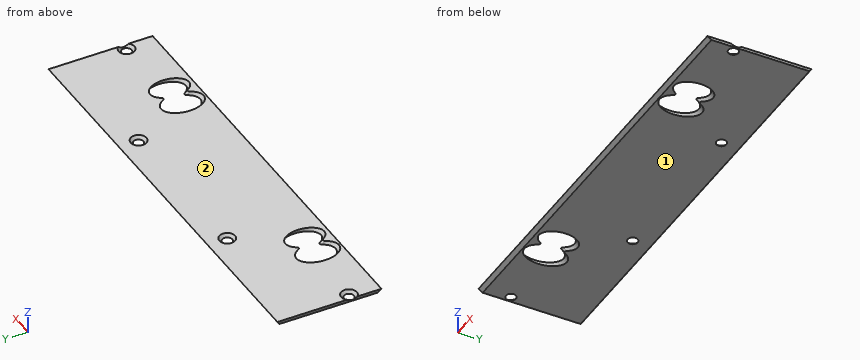
Autodesk Inventor part; units mm, degrees
ref_plane "Work Plane2" through (178, -42.7329, -77.104) normal (1, 0, 0) x (0, 0.819152, -0.5735764)
ref_plane "YZ Plane" through (0, 0, 0) normal (1, 0, 0) x (0, 1, 0)
ref_plane "XZ Plane" through (0, 0, 0) normal (0, 1, 0) x (-1, 0, 0)
ref_plane "Work Plane1" through (0, -45.8455, -0.8595) normal (-1, 0, 0) x (0, 0.5735764, 0.819152)
sketch "Sketch1" plane through (0, -45.8455, -0.8595) normal (-1, 0, 0) x (0, 0.5735764, 0.819152)
  line L0 (4.2002, 4.5) -> (27, 37.0615)
  line L1 (3.5, -0.5) -> (3.5, 3.5)
  line L2 (27, 37.0615) -> (28, 37.0615)
  line L3 (27, 37.0615) -> (3.5, 3.5)
  line L4 (3.5, 1.4079) -> (28.4649, 37.0615)
  line L5 (27, 37.0615) -> (28.4649, 37.0615)
  point P0 (4.2002, 4.5)
  dimension "d0" = 1.2
  dimension "d1" = 55
ref_plane "Work Plane2" through (178, -42.7329, -77.104) normal (1, 0, 0) x (0, 0.819152, -0.5735764)
extrude "Extrusion1" add sketch "Sketch1" against normal up to surface (178 mm away)
ref_plane "Work Plane3" through (36.3849, -23.4357, -7.1547) normal (0, -0.7489557, 0.66262) x (1, 0, 0)
ref_plane "Work Plane4" through (36.3849, -23.4357, -7.1547) normal (0, -0.7489557, 0.66262) x (1, 0, 0)
sketch "Sketch4" plane through (36.3849, -23.4357, -7.1547) normal (0, -0.7489557, 0.66262) x (1, 0, 0)
  line L0 (-14.9215, 5.4518) -> (-14.9215, -5.4534)
  spline S0 degree 3 poles (-14.9215, -5.4534) (-14.9222, -5.5772) (-14.8715, -5.6989) (-14.7851, -5.7853) (-14.7653, -5.8051) (-14.7437, -5.823) (-14.7206, -5.8388) (-14.7012, -5.8521) (-14.6808, -5.864) (-14.6595, -5.8743) (-14.6436, -5.882) (-14.6272, -5.8889) (-14.6105, -5.8948) (-14.5603, -5.9125) (-14.5071, -5.9218) (-14.4534, -5.9215) knots 0 0 0 0 0.5 0.5 0.5 0.614375 0.614375 0.614375 0.710781 0.710781 0.710781 0.783086 0.783086 0.783086 1 1 1 1
  line L1 (-14.4534, -5.9215) -> (14.4534, -5.9215)
  spline S1 degree 3 poles (14.4534, -5.9215) (14.5775, -5.9222) (14.6994, -5.8713) (14.8723, -5.6977) (14.9222, -5.5758) (14.9215, -5.4518) knots 0 0 0 0 0.5 0.5 1 1 1 1
  line L2 (14.9215, -5.4518) -> (14.9215, 5.4534)
  spline S2 degree 3 poles (14.9215, 5.4534) (14.9222, 5.5775) (14.8713, 5.6994) (14.6977, 5.8723) (14.5758, 5.9222) (14.4518, 5.9215) knots 0 0 0 0 0.5 0.5 1 1 1 1
  line L3 (14.4518, 5.9215) -> (-14.4534, 5.9215)
  spline S3 degree 3 poles (-14.4534, 5.9215) (-14.5775, 5.9222) (-14.6994, 5.8713) (-14.8723, 5.6977) (-14.9222, 5.5758) (-14.9215, 5.4518) knots 0 0 0 0 0.5 0.5 1 1 1 1
  circle A0 centre (-13.3791, -4.3791) radius 0.5
  circle A1 centre (-13.3791, 4.3791) radius 0.5
  circle A2 centre (13.3791, 4.3791) radius 0.5
  circle A3 centre (13.3791, -4.3791) radius 0.5
  arc A4 (0.2617, -1.4512) -> (0.1811, -1.5218) centre (0.2771, -1.55) ccw
  arc A5 (0.1811, 1.5218) -> (0.1811, -1.5218) centre (-5, 0) ccw
  arc A6 (0.1811, 1.5218) -> (0.2617, 1.4512) centre (0.2771, 1.55) ccw
  arc A7 (0.2617, 1.4512) -> (0.3414, 1.519) centre (0.2463, 1.55) ccw
  arc A8 (0.3414, -1.519) -> (0.3414, 1.519) centre (5, 0) ccw
  arc A9 (0.3414, -1.519) -> (0.2617, -1.4512) centre (0.2463, -1.55) ccw
  line L4 (90.3087, 5.4518) -> (90.3087, -5.4534)
  spline S4 degree 3 poles (90.3087, -5.4534) (90.308, -5.5772) (90.3587, -5.6989) (90.4451, -5.7853) (90.4649, -5.8051) (90.4865, -5.823) (90.5096, -5.8388) (90.529, -5.8521) (90.5494, -5.864) (90.5707, -5.8743) (90.5866, -5.882) (90.603, -5.8889) (90.6197, -5.8948) (90.6699, -5.9125) (90.7231, -5.9218) (90.7769, -5.9215) knots 0 0 0 0 0.5 0.5 0.5 0.614375 0.614375 0.614375 0.710781 0.710781 0.710781 0.783086 0.783086 0.783086 1 1 1 1
  line L5 (90.7769, -5.9215) -> (119.6836, -5.9215)
  spline S5 degree 3 poles (119.6836, -5.9215) (119.8077, -5.9222) (119.9296, -5.8713) (120.1025, -5.6977) (120.1524, -5.5758) (120.1517, -5.4518) knots 0 0 0 0 0.5 0.5 1 1 1 1
  line L6 (120.1517, -5.4518) -> (120.1517, 5.4534)
  spline S6 degree 3 poles (120.1517, 5.4534) (120.1524, 5.5775) (120.1015, 5.6994) (119.9279, 5.8723) (119.806, 5.9222) (119.682, 5.9215) knots 0 0 0 0 0.5 0.5 1 1 1 1
  line L7 (119.682, 5.9215) -> (90.7769, 5.9215)
  spline S7 degree 3 poles (90.7769, 5.9215) (90.6527, 5.9222) (90.5308, 5.8713) (90.3579, 5.6977) (90.308, 5.5758) (90.3087, 5.4518) knots 0 0 0 0 0.5 0.5 1 1 1 1
  circle A10 centre (91.8511, -4.3791) radius 0.5
  circle A11 centre (91.8511, 4.3791) radius 0.5
  circle A12 centre (118.6093, 4.3791) radius 0.5
  circle A13 centre (118.6093, -4.3791) radius 0.5
  arc A14 (105.4919, -1.4512) -> (105.4113, -1.5218) centre (105.5073, -1.55) ccw
  arc A15 (105.4113, 1.5218) -> (105.4113, -1.5218) centre (100.2302, 0) ccw
  arc A16 (105.4113, 1.5218) -> (105.4919, 1.4512) centre (105.5073, 1.55) ccw
  arc A17 (105.4919, 1.4512) -> (105.5716, 1.519) centre (105.4765, 1.55) ccw
  arc A18 (105.5716, -1.519) -> (105.5716, 1.519) centre (110.2302, 0) ccw
  arc A19 (105.5716, -1.519) -> (105.4919, -1.4512) centre (105.4765, -1.55) ccw
  arc A20 (105.5127, 2.6278) -> (105.5127, -2.6278) centre (100.2302, 0) ccw
  arc A21 (105.5127, -2.6278) -> (105.5127, 2.6278) centre (110.2302, 0) ccw
  arc A22 (0.2825, 2.6278) -> (0.2825, -2.6278) centre (-5, 0) ccw
  arc A23 (0.2825, -2.6278) -> (0.2825, 2.6278) centre (5, 0) ccw
  point P0 (-36.3849, 20.8875)
  dimension "d27" = 0.5
  dimension "d28" = 0.5
extrude "Extrusion2" cut sketch "Sketch4" along normal up to next contours A4 A5 A6 A7 A8 A9 | A14 A15 A16 A17 A18 A19 | A21 A20 | A23 A22
sketch "Sketch6" plane through (0, -42.6848, 1.2) normal (0, 0, 1) x (1, 0, 0)
  circle A0 centre (54.5, 35.1848) radius 2.3
  circle A1 centre (123.5, 35.1848) radius 2.3
  circle A2 centre (2.5, 12.2262) radius 2.3
  circle A3 centre (175.5, 12.2262) radius 2.3
  point P0 (0, 42.6848)
hole "Hole1" at (54.5, -7.5, 1.2) at (123.5, -7.5, 1.2) at (2.5, -30.4585, 1.2) at (175.5, -30.4585, 1.2) direction (0, 0, -1) diameter 3.6 end through all countersink diameter 6.6 countersink angle 90
fillet "Fillet1" radius 1 4 edges at (36.6674, -36.1666, 0.6) (36.6674, -28.2351, 0.6) (141.8976, -28.2351, 0.6) (141.8976, -36.1666, 0.6)
properties part number "front" material "Nylon 6/6"
Input: part model. Units: mm. Frame: model coordinates. Face numbers are marked on the shaded views. Coordinates: 2 decimals unless noted, no trailing zeros. Write each loop counter-clockwise with the first axis right and the second up, starting at its lowest first coordinate (ties: lowest second). Pieces come first, ordered by that corner, then holes. Notation, with made-up numbers: (73, -18.75) -> (122, -18.75) arc R12 ccw to (122, -13.75) -> close; hole circle Ø4 at (32, 81.25). An arc over 180 degrees is marked (long way). Answer as a JSON object with one key per item and string values.
1. Material intervals for line 1 (X direction, y = -6, z = 0.5); line 2 (X direction, y = -6, z = 0.85); line 3 (X direction, y = -28, z = 0.9), sorted ascending. Write a range as from..to.
Result set:
{"line 1": "x = 0..52.38, 56.62..121.38, 125.62..178", "line 2": "x = 0..51.96, 57.04..120.96, 126.04..178", "line 3": "x = 0..0.78, 4.22..26.31, 45.87..131.54, 151.1..173.78, 177.22..178"}
2. Mould query, pull axis Z, two halves, no side actions, for the marked faces 1 and 2. Classes: released by +Z, released by -Z, zero draft, split by the parting line, or undercut.
Result set:
{"face 1": "released by -Z", "face 2": "released by +Z"}
3. Section C-C on z = 1. Count the separate pieces of the cut face and the enclosed holes in it, then the cut area to 3 significant figures.
Result set:
{"separate pieces": "1", "enclosed holes": "4", "area": "6,960 mm2"}
4. Section B-B on y = -7.5. Return the cut outline in (x, z), then the cut area to 3 significant figures.
Result set:
{"outline": "(0, 0) -> (52.4, 0) -> (51.2, 1.2) -> (0, 1.2) -> close; (56.6, 0) -> (121.4, 0) -> (120.2, 1.2) -> (57.8, 1.2) -> close; (125.6, 0) -> (178, 0) -> (178, 1.2) -> (126.8, 1.2) -> close", "area": "201 mm2"}
5. Section A-A on x = 2.5. Return the cut outline in (y, z).
Result set:
{"outline": "(-42.68, 1.2) -> (-40.97, 0) -> (-32.56, 0) -> (-33.76, 1.2) -> close; (-28.36, 0) -> (0, 0) -> (0.84, 1.2) -> (-27.16, 1.2) -> close"}
6. Section D-D on x = 83. Return the cut outline in (y, z), then the cut area to 3 significant figures.
Result set:
{"outline": "(-42.68, 1.2) -> (-40.97, 0) -> (0, 0) -> (0.84, 1.2) -> close", "area": "50.7 mm2"}
